The drawing under review shows one solid part. Ordinate dimensions are in mm from its lowest x, y, z. A direction names the side the tool comes from. Give positions to 0.01 mm unless a question says otherwise; leave off trailing zeros. Write each loop counter-clockwise with the first axis right and the second up, starting at its lowest first coordinate (ties: lowest second). Pieces come first, ordered by that corner, then holes. Notation, with made-up numbers: M 14.25,-20.5 L 39.25,-20.5 A23 cw 39.25,18.5 Z; hole C -13,-21 d4. An arc over 180 degrees is marked long. One line per item, written item: value. Start each with the question number.
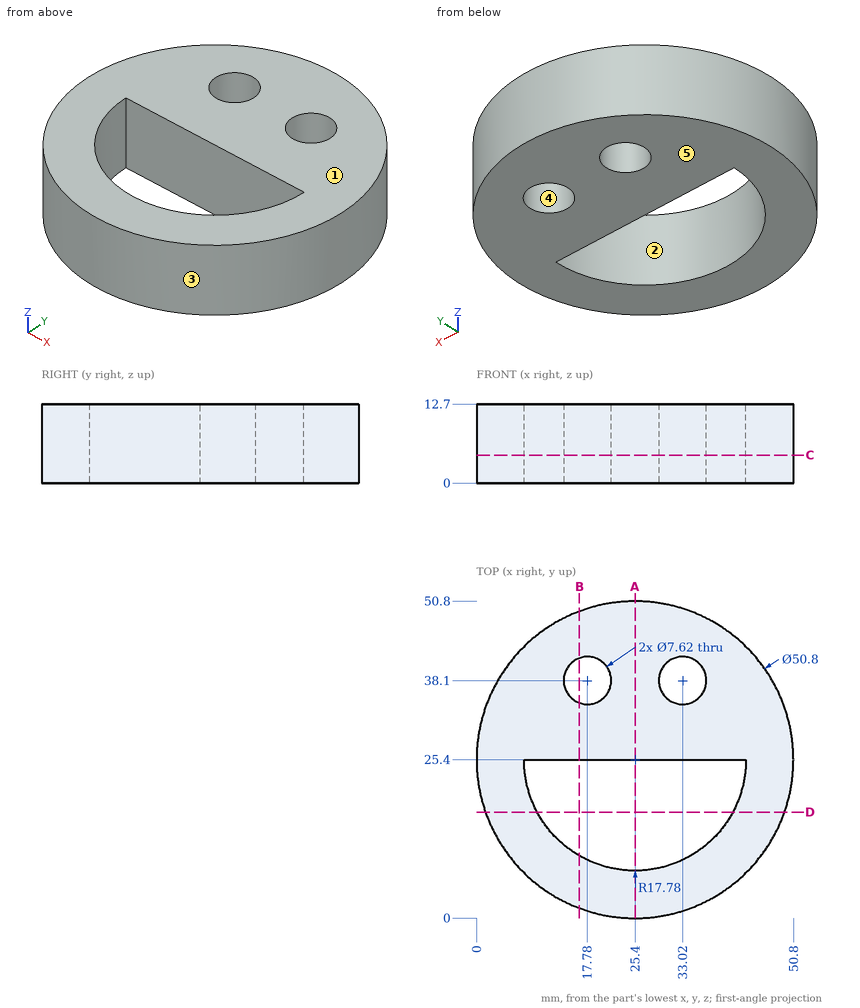
Q1. The part is to be moulded in two halves that separate along X. For the marked faces 3, 4 and 5, say which applies: pulls with the +X half, pulls with the -X half, needs draft (parallel to the pull), parting line crosses it, or undercut.
Q2. For P1, Ø1, axis at x = 35, y = 35, coming from the -Z side; P2, Ø6, axis at y = 18, z = 8, coming from the +X side; P3, Ø1, axis at y = 11, z = 5.5, coming from the +X side; P4, Ø3, axis at y = 18.5, z = 3.5, coming from the +X side, all flat-tipped, find the tip position at first contact; note any pin that passes through.
Q3. Machinability: for the marked faces 1 and 2, which of the approach directions +Z, -Z, +X, -X, +Y, -Y give a long, thin tool a straight path to every point of the face, cutting with its end or side? Answer none if there is none.
Q4. Wall thickness on line 1 (Y direction, x = 32, z = 10.75); line 2 (Y direction, x = 17.78, z = 8.5); line 3 (X direction, y = 9.5, z = 3): over which ranges is each line inside the solid? List them lowest first. Write a range as from..to.
Q5. Take a section at B-B, the plane x = 16.5. Give the boundary of the cut face in (y, z).
Q6. Take a section at A-A, the plane x = 25.4. Give the boundary of the cut face in (y, z).
Q7. Take a section at C-C, the plane z = 4.5. Give the boundary of the cut face in (x, y).
Q8. Take a section at D-D, the plane y = 17. Give the boundary of the cut face in (x, z).
Results list:
1. face 3: parting line crosses it
1. face 4: undercut
1. face 5: needs draft
2. P1: stops at z = 0
2. P2: stops at x = 50.42
2. P3: stops at x = 46.66
2. P4: stops at x = 50.22
3. face 1: +Z, +X, -X, +Y, -Y
3. face 2: +Z, -Z
4. line 1: y = 0.87..8.89, 25.4..34.43, 41.77..49.93
4. line 2: y = 1.17..9.34, 25.4..34.29, 41.91..49.63
4. line 3: x = 5.59..17.44, 33.36..45.21
5. outline: M 1.61,0 L 10.01,0 L 10.01,12.7 L 1.61,12.7 Z; M 25.4,0 L 34.51,0 L 34.51,12.7 L 25.4,12.7 Z; M 41.69,0 L 49.19,0 L 49.19,12.7 L 41.69,12.7 Z
6. outline: M 0,0 L 7.62,0 L 7.62,12.7 L 0,12.7 Z; M 25.4,0 L 50.8,0 L 50.8,12.7 L 25.4,12.7 Z
7. outline: C 25.4,25.4 d50.8; hole M 7.62,25.4 A17.78 ccw 43.18,25.4 Z; hole C 17.78,38.1 d7.62; hole C 33.02,38.1 d7.62
8. outline: M 1.43,0 L 9.73,0 L 9.73,12.7 L 1.43,12.7 Z; M 41.07,0 L 49.37,0 L 49.37,12.7 L 41.07,12.7 Z
